Geometry: final body of the model. Coordinates: model frame, mm. Face numbers are marked on the shaded views. A direction names the side the tool comes from. Round coordinates to 2 decimals unless told otherwise and drop trailing zeros. Order: outer loops, then holes, each group sorted by start corner. A loop starts at its lowest first (then second) coordinate and runs counter-clockwise, first axis right, second up. Notation, with made-up numbers: M 3,46 L 33,46 A12 cw 33,66 Z; hole C -5,52.25 d1. An arc over 180 degrees is marked long. Put each result on its own line as item: value. Start each with the question number.
1) Section A-A, the plane x = -5.5. Return loops of the section in (y, z), then the cut area to 3 significant figures.
2) First-contact query: P1, Ø2.5, axis at x = 8, z = 5, coming from the +Y side. Flat tip, straight axial feed; report the tip coordinate or a pass-through.
3) Section B-B, the plane z = 1.75. Return loops of the section in (x, y), then the cut area to 3 significant figures.
4) Draft query along X for the marked faces 3, 4 and 5. Return one class per face: pulls with the +X half, pulls with the -X half, needs draft (parallel to the pull), parting line crosses it, or undercut.
5) Access query for the marked faces 1 and 2. Directions: +Z, -Z, +X, -X, +Y, -Y. A direction counts if a zero-diameter tool reaches every point of the face in a straight line with its end or side. Return the directions, or none.
6) Material intervals for probe 1 along X at (y, z) = (13, 2); probe 2 along X at (y, z) = (15.25, 4.75); probe 3 along Y at (x, z) = (9.5, 5), sorted ascending. Write a range as [from, to].
7) Section C-C, the plane x = -17.5. Return loops of the section in (y, z), then the cut area to 4 significant figures.
from build123d import *

# Parameters (mm, degrees)
PAD_DEPTH       = 7
SKETCH001_W     = 65
SKETCH001_H     = 1.8
POCKET_DEPTH    = 3.5
CHAMFER_SIZE    = 0.5
CHAMFER001_SIZE = 0.5


with BuildPart() as part:
    # Sketch → Pad (new body)
    with BuildSketch(Plane.XY):
        Polygon((-32.5, 0), (-32.5, 15.8), (-27.5, 15.8), (-27.5, 13.8), (-29.5, 13.8), (-29.5, 12), (-27.5, 12), (-27.5, 10), (-6.5, 10), (-6.5, 12), (-4.5, 12), (-4.5, 13.8), (-6.5, 13.8), (-6.5, 15.8), (6.5, 15.8), (6.5, 13.8), (4.5, 13.8), (4.5, 12), (6.5, 12), (6.5, 10), (27.5, 10), (27.5, 12), (29.5, 12), (29.5, 13.8), (27.5, 13.8), (27.5, 15.8), (32.5, 15.8), (32.5, 0), align=None)
    extrude(amount=PAD_DEPTH)

    # Sketch001 → Pocket (cut)
    with BuildSketch(Plane.XY.offset(7)):
        with Locations((0, 2.9)):
            Rectangle(SKETCH001_W, SKETCH001_H)
    extrude(amount=-POCKET_DEPTH, mode=Mode.SUBTRACT)

    # Chamfer
    chamfer_edges = [part.edges().sort_by_distance(p)[0] for p in [
        (0, 2, 7),
        (0, 3.8, 7),
        (-32.5, 2, 5.25),
        (-32.5, 3.8, 5.25),
        (32.5, 2, 5.25),
        (32.5, 3.8, 5.25),
    ]]
    chamfer(chamfer_edges, length=CHAMFER_SIZE)

    # Chamfer001
    chamfer001_edges = [part.edges().sort_by_distance(p)[0] for p in [
        (-28.5, 12, 7),
        (-28.5, 13.8, 7),
        (-5.5, 12, 7),
        (-5.5, 13.8, 7),
        (5.5, 12, 7),
        (5.5, 13.8, 7),
        (28.5, 12, 7),
        (28.5, 13.8, 7),
    ]]
    chamfer(chamfer001_edges, length=CHAMFER001_SIZE)


solid = part.part
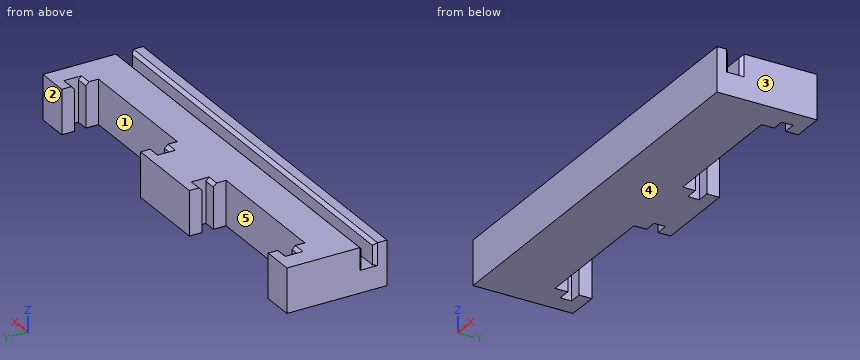
Result sheet:
1. outline: M 0,0 L 12,0 L 12,6.5 L 11.5,7 L 4.3,7 L 3.8,6.5 L 3.8,3.5 L 2,3.5 L 2,6.5 L 1.5,7 L 0,7 Z; M 13.8,0 L 15.8,0 L 15.8,7 L 14.3,7 L 13.8,6.5 Z
1. area: 91.2 mm2
2. P1: stops at y = 10
3. outline: M -32.5,0 L 32.5,0 L 32.5,15.8 L 27.5,15.8 L 27.5,13.8 L 29.5,13.8 L 29.5,12 L 27.5,12 L 27.5,10 L 6.5,10 L 6.5,12 L 4.5,12 L 4.5,13.8 L 6.5,13.8 L 6.5,15.8 L -6.5,15.8 L -6.5,13.8 L -4.5,13.8 L -4.5,12 L -6.5,12 L -6.5,10 L -27.5,10 L -27.5,12 L -29.5,12 L -29.5,13.8 L -27.5,13.8 L -27.5,15.8 L -32.5,15.8 Z
3. area: 769 mm2
4. face 3: pulls with the +X half
4. face 4: needs draft
4. face 5: undercut
5. face 1: +Z, -Z, +Y
5. face 2: +Z, -Z, +X, -X, +Y
6. probe 1: x = [-32.5, -29.5], [-4.5, 4.5], [29.5, 32.5]
6. probe 2: x = [-32.5, -27.5], [-6.5, 6.5], [27.5, 32.5]
6. probe 3: y = [0, 2], [3.8, 10]
7. outline: M 0,0 L 10,0 L 10,7 L 4.3,7 L 3.8,6.5 L 3.8,3.5 L 2,3.5 L 2,6.5 L 1.5,7 L 0,7 Z
7. area: 63.45 mm2
